```python
from build123d import *

# Parameters (mm, degrees)
SKETCH_1_W             = 900
SKETCH_1_H             = 680
EXTRUDE_1_DEPTH        = 40
SKETCH_2_W             = 50
SKETCH_2_H             = 340
CUT_EXTRUDE_1_DEPTH    = 566.420197729
HOLE_WIZARD_M5_1_D     = 4.2
HOLE_WIZARD_M5_2_D     = 4.2
SKETCH_9_R             = 12.5
CUT_EXTRUDE_2_DEPTH    = 566.420197876
HOLE_WIZARD_M5_3_D     = 4.2
HOLE_WIZARD_M5_3_DEPTH = 5.2
HOLE_WIZARD_M5_3_TIP   = 1.2618073
HOLE_WIZARD_M3_1_D     = 2.5
HOLE_WIZARD_M3_1_DEPTH = 8.5
HOLE_WIZARD_M3_1_TIP   = 0.751075774


with BuildPart() as part:
    # 草图1 → 凸台-拉伸1 (new body)
    with BuildSketch(Plane(origin=(0, 0, 0), x_dir=(1, 0, 0), z_dir=(0, 1, 0))):
        Rectangle(SKETCH_1_W, SKETCH_1_H)
    extrude(amount=EXTRUDE_1_DEPTH)

    # 草图2 → 切除-拉伸1 (cut, through all)
    with BuildSketch(Plane(origin=(0, 40, 0), x_dir=(1, 0, 0), z_dir=(0, 1, 0))):
        with BuildLine():
            Line((-25, -8), (-25, -158))
            ThreePointArc((-25, -158), (60, -243), (145, -158))
            Line((145, -158), (145, -8))
            ThreePointArc((145, -8), (60, 77), (-25, -8))
        make_face()
        with BuildLine():
            Line((-225, -8), (-225, -158))
            ThreePointArc((-225, -158), (-140, -243), (-55, -158))
            Line((-55, -158), (-55, -8))
            ThreePointArc((-55, -8), (-140, 77), (-225, -8))
        make_face()
        with Locations((210, -83)):
            Rectangle(SKETCH_2_W, SKETCH_2_H)
    extrude(amount=-CUT_EXTRUDE_1_DEPTH, mode=Mode.SUBTRACT)

    # M5 螺纹孔1 (through all)
    with Locations(Plane.XY.offset(340)):
        with Locations((0, 20)):
            Hole(HOLE_WIZARD_M5_1_D / 2)

    # M5 螺纹孔2 (through all)
    with Locations(Plane.ZY.offset(450)):
        with Locations((0, 20)):
            Hole(HOLE_WIZARD_M5_2_D / 2)

    # 草图9 → 切除-拉伸2 (cut, through all)
    with BuildSketch(Plane(origin=(0, 40, 0), x_dir=(1, 0, 0), z_dir=(0, 1, 0))):
        with Locations(Location((-398, 250, 0), (0, 0, 270))):
            Circle(SKETCH_9_R)
    extrude(amount=-CUT_EXTRUDE_2_DEPTH, mode=Mode.SUBTRACT)

    # M5 螺纹孔3
    with Locations(Plane(origin=(0, 40, 0), x_dir=(1, 0, 0), z_dir=(0, 1, 0))):
        with Locations((-295, -31.1), (-295, -81.1), (315, -31.1), (315, -81.1)):
            Hole(HOLE_WIZARD_M5_3_D / 2, depth=HOLE_WIZARD_M5_3_DEPTH)
            with Locations((0, 0, -(HOLE_WIZARD_M5_3_DEPTH + HOLE_WIZARD_M5_3_TIP / 2))):  # 118° drill point
                Cone(0, HOLE_WIZARD_M5_3_D / 2, HOLE_WIZARD_M5_3_TIP, mode=Mode.SUBTRACT)

    # M3 螺纹孔1
    with Locations(Plane(origin=(0, 40, 0), x_dir=(1, 0, 0), z_dir=(0, 1, 0))):
        with Locations((-289.5, 304.5), (-264.5, 304.5), (-264.5, 279.5), (-289.5, 279.5), (255.8, 304.5), (255.8, 279.5), (230.8, 279.5), (230.8, 304.5)):
            Hole(HOLE_WIZARD_M3_1_D / 2, depth=HOLE_WIZARD_M3_1_DEPTH)
            with Locations((0, 0, -(HOLE_WIZARD_M3_1_DEPTH + HOLE_WIZARD_M3_1_TIP / 2))):  # 118° drill point
                Cone(0, HOLE_WIZARD_M3_1_D / 2, HOLE_WIZARD_M3_1_TIP, mode=Mode.SUBTRACT)


solid = part.part
```
Read the model definition and answer for the solid it produces. Units are mm, in the model's axes. A direction names the side the tool comes from. Give positions to 0.01 mm unless a question says otherwise; leave off trailing zeros. Loops run counter-clockwise (first coordinate to the right, second up) from the corner with the lowest first, then second, coordinate; pieces in that order, holes last.
Item 1: The mould has two halves that part along X. Classify faces 3 (the flat face through (-450, 20, 5)), 4 (the flat face through (-6, 20, 340)), 5 (the flat face through (235, 20, 85)), 6 (the cylindrical face through (58.13, 20.28, 242.98)): released by +X, released by -X, zero draft, split by the parting line, or undercut.
Item 2: The part is cut by section B-B (x = 60). Write down the section's boundary in (y, z), and give its area (3 significant figures).
Item 3: The part is cut by section A-A (y = 6.5). Write down the section's boundary in (x, z).
Item 4: This flat-tipped pin is pushed along its axis until it touches: pin 1 Ø1.5 at (x, z) = (230.8, -279.5) entering from +Y. Where does it stop, or does it pass through?
Item 5: Find the intervals of material crossed by line 1 along X through (y, z) = (36, 31); line 2 along X through (y, z) = (31, 146.5); line 3 along Z through (x, y) = (-295, 38.1), in increasing order.
Item 6: For faces 1 (the flat face through (-55, 20, 84)), 2 (the flat face through (-6, 40, -80)), determine the directions among +Z, -Z, +X, -X, +Y, -Y from which every point of the face is accessible in a straight line to the end or side of a thin tool.
Item 7: The part is cut by section C-C (x = -90.5). Write down the section's boundary in (y, z), and give its area (3 significant figures).
Taken from the geometry:
1. face 3: released by -X
1. face 4: zero draft
1. face 5: undercut
1. face 6: undercut
2. outline: (0, -340) - (40, -340) - (40, -77) - (0, -77) - close; (0, 243) - (40, 243) - (40, 340) - (0, 340) - close
2. area: 14,400 mm2
3. outline: (-450, -340) - (450, -340) - (450, 340) - (-450, 340) - close; hole circle Ø25 at (-398, -250); hole (-225, 8) arc R85 ccw to (-55, 8) - (-55, 158) arc R85 ccw to (-225, 158) - close; hole (-25, 8) arc R85 ccw to (145, 8) - (145, 158) arc R85 ccw to (-25, 158) - close; hole (185, -87) - (235, -87) - (235, 253) - (185, 253) - close
4. pin 1: stops at y = 31.2
5. line 1: x = -450 to -297.1, -292.9 to -225, -55 to -25, 145 to 185, 235 to 312.9, 317.1 to 450
5. line 2: x = -450 to -225, -55 to -25, 145 to 185, 235 to 450
5. line 3: z = -340 to 29, 33.2 to 79, 83.2 to 340
6. face 1: +Y, -Y
6. face 2: +Z, -Z, +X, -X, +Y
7. outline: (0, -340) - (40, -340) - (40, -61.1) - (0, -61.1) - close; (0, 227.1) - (40, 227.1) - (40, 340) - (0, 340) - close
7. area: 15,700 mm2
